Input: part model. Units: mm. Frame: model coordinates. A direction names the side the tool comes from. Round coordinates to 2 decimals unless told otherwise and drop trailing zeros. Order: outer loops, then holes, each group sorted by start corner. A loop starts at its lowest first (then second) coordinate and runs counter-clockwise, first axis right, second up. Notation, with made-up numbers: (-30, 0.25) - (-14, 0.25) arc R18 cw to (-14, 10.25) - close; hole circle Ø10 at (-8, 89.5). An arc over 180 degrees is marked (long way). One line per item, written item: value. Start each with the question number.
from build123d import *

# Parameters (mm, degrees)
SKETCH1_W           = 59
SKETCH1_H           = 68
SKETCH1_R           = 1
SKETCH1_R_2         = 1.5
BOSS_EXTRUDE1_DEPTH = 2
FILLET1_R           = 5
CUT_EXTRUDE1_DEPTH  = 2
SKETCH3_R           = 3
SKETCH3_R_2         = 1
BOSS_EXTRUDE2_DEPTH = 4


with BuildPart() as part:
    # Sketch1 → Boss-Extrude1 (new body)
    with BuildSketch(Plane(origin=(0, 0, 0), x_dir=(1, 0, 0), z_dir=(0, 1, 0))):
        with Locations((29.5, 34)):
            Rectangle(SKETCH1_W, SKETCH1_H)
        with Locations(Location((5, 5, 0), (0, 0, 270))):
            Circle(SKETCH1_R, mode=Mode.SUBTRACT)
        with Locations(Location((54, 5, 0), (0, 0, 270))):
            Circle(SKETCH1_R, mode=Mode.SUBTRACT)
        with Locations(Location((5, 63, 0), (0, 0, 270))):
            Circle(SKETCH1_R, mode=Mode.SUBTRACT)
        with Locations(Location((54, 63, 0), (0, 0, 270))):
            Circle(SKETCH1_R, mode=Mode.SUBTRACT)
        with Locations(Location((9.5, 59, 0), (0, 0, 270))):
            Circle(SKETCH1_R_2, mode=Mode.SUBTRACT)
        with Locations(Location((49.5, 59, 0), (0, 0, 270))):
            Circle(SKETCH1_R_2, mode=Mode.SUBTRACT)
        with Locations(Location((49.5, 9, 0), (0, 0, 270))):
            Circle(SKETCH1_R_2, mode=Mode.SUBTRACT)
        with Locations(Location((9.5, 9, 0), (0, 0, 270))):
            Circle(SKETCH1_R_2, mode=Mode.SUBTRACT)
    extrude(amount=BOSS_EXTRUDE1_DEPTH)

    # Fillet1
    fillet1_edges = [part.edges().sort_by_distance(p)[0] for p in [
        (0, 1, -68),
        (59, 1, -68),
        (59, 1, 0),
        (0, 1, 0),
    ]]
    fillet(fillet1_edges, radius=FILLET1_R)

    # Sketch2 → Cut-Extrude1 (cut)
    with BuildSketch(Plane(origin=(0, 2, 0), x_dir=(1, 0, 0), z_dir=(0, 1, 0))):
        with BuildLine():
            Line((0, 5), (18.940260842, 27.572123903))
            ThreePointArc((18.940260842, 27.572123903), (21.279816411, 34), (18.940260842, 40.427876097))
            Line((18.940260842, 40.427876097), (0, 63))
            Line((0, 63), (0, 5))
        make_face()
        with BuildLine():
            Line((54, 0), (36.255902076, 16.259470082))
            ThreePointArc((36.255902076, 16.259470082), (29.5, 18.886696714), (22.744097924, 16.259470082))
            Line((22.744097924, 16.259470082), (5, 0))
            Line((5, 0), (54, 0))
        make_face()
        with BuildLine():
            Line((54, 68), (5, 68))
            Line((5, 68), (22.744097924, 51.740529918))
            ThreePointArc((22.744097924, 51.740529918), (29.5, 49.113303286), (36.255902076, 51.740529918))
            Line((36.255902076, 51.740529918), (54, 68))
        make_face()
        with BuildLine():
            Line((59, 5), (59, 63))
            Line((59, 63), (40.059739158, 40.427876097))
            ThreePointArc((40.059739158, 40.427876097), (37.720183589, 34), (40.059739158, 27.572123903))
            Line((40.059739158, 27.572123903), (59, 5))
        make_face()
    extrude(amount=-CUT_EXTRUDE1_DEPTH, mode=Mode.SUBTRACT)

    # Sketch3 → Boss-Extrude2 (add)
    # profile 1 of 4: a face of its own
    with BuildSketch(Plane(origin=(0, 2, 0), x_dir=(1, 0, 0), z_dir=(0, 1, 0))):
        with Locations(Location((5, 63, 0), (0, 0, 270))):
            Circle(SKETCH3_R)
        with Locations(Location((5, 63, 0), (0, 0, 270))):
            Circle(SKETCH3_R_2, mode=Mode.SUBTRACT)
    # profile 2 of 4: a face of its own
    with BuildSketch(Plane(origin=(0, 2, 0), x_dir=(1, 0, 0), z_dir=(0, 1, 0))):
        with Locations(Location((54, 63, 0), (0, 0, 90))):
            Circle(SKETCH3_R)
        with Locations(Location((54, 63, 0), (0, 0, 270))):
            Circle(SKETCH3_R_2, mode=Mode.SUBTRACT)
    # profile 3 of 4: a face of its own
    with BuildSketch(Plane(origin=(0, 2, 0), x_dir=(1, 0, 0), z_dir=(0, 1, 0))):
        with Locations(Location((54, 5, 0), (0, 0, 90))):
            Circle(SKETCH3_R)
        with Locations(Location((54, 5, 0), (0, 0, 270))):
            Circle(SKETCH3_R_2, mode=Mode.SUBTRACT)
    # profile 4 of 4: a face of its own
    with BuildSketch(Plane(origin=(0, 2, 0), x_dir=(1, 0, 0), z_dir=(0, 1, 0))):
        with Locations(Location((5, 5, 0), (0, 0, 90))):
            Circle(SKETCH3_R)
        with Locations(Location((5, 5, 0), (0, 0, 270))):
            Circle(SKETCH3_R_2, mode=Mode.SUBTRACT)
    extrude(amount=BOSS_EXTRUDE2_DEPTH)


solid = part.part
1. Line query: line 1 (X direction, y = 4.2, z = -63); line 2 (X direction, y = 0.75, z = -9); line 3 (Y direction, x = 44, z = -50). Output: solid intervals per line, ascending. Write a range as from..to.
2. Section A-A (y = 3.3). Return the cut outline in (x, z).
3. Section C-C (z = -54). Return the cut outline in (x, y), then the cut area to 3 significant figures.
4. Pin query (flat end, axial travel): pin 1 (3.5 mm diameter, centred on x = 9.5, z = -59, fed in from +Y); pin 2 (1.5 mm diameter, centred on x = 43.5, y = 2.5, fed in from -Z). Return the tip coordinate at first contact, or that it passes through.
5. Pull-direction query (X, two-part tool) for faces 1 (the face through (6.8, 4, -2.6)), 2 (the face through (9.34, 1.01, -16.13)), 3 (the face through (53, 6, -4)); classes: released by +X, released by -X, zero draft, split by the parting line, or undercut.
6. Section D-D (x = 43.5). Return the cut outline in (y, z).
7. Set-up query: faces 4 (the face through (9.6, 1.01, -51.56)), 5 (the face through (45.004, 1.014, -59.756)), 6 (the face through (13.996, 1.014, -8.244)), 7 (the face through (51, 4, -5)). Return all of +Z, -Z, +X, -X, +Y, -Y with unobstructed straight access to the full face (end or side cutting, diameter ignored); none if empty.
8. Section B-B (x = 9.5). Return the cut outline in (y, z), then the cut area to 3 significant figures.
Solved:
1. line 1: x = 2..4, 6..8, 51..53, 55..57
1. line 2: x = 3.36..8, 11..14.82, 44.18..48, 51..55.64
1. line 3: y = 0..2
2. outline: circle Ø6 at (5, -63); circle Ø6 at (5, -5); circle Ø6 at (54, -63); circle Ø6 at (54, -5); hole circle Ø2 at (5, -63); hole circle Ø2 at (5, -5); hole circle Ø2 at (54, -63); hole circle Ø2 at (54, -5)
3. outline: (7.55, 0) - (20.28, 0) - (20.28, 2) - (7.55, 2) - close; (38.72, 0) - (51.45, 0) - (51.45, 2) - (38.72, 2) - close
3. area: 50.9 mm²
4. pin 1: stops at y = 2
4. pin 2: stops at z = -58.89
5. face 1: undercut
5. face 2: released by -X
5. face 3: zero draft
6. outline: (0, -58.38) - (2, -58.38) - (2, -44.53) - (0, -44.53) - close; (0, -23.47) - (2, -23.47) - (2, -9.62) - (0, -9.62) - close
7. face 4: -X, +Y, -Y
7. face 5: -Z, +Y, -Y
7. face 6: +Z, +Y, -Y
7. face 7: +Y
8. outline: (0, -63.88) - (2, -63.88) - (2, -60.5) - (0, -60.5) - close; (0, -57.5) - (2, -57.5) - (2, -51.68) - (0, -51.68) - close; (0, -16.32) - (2, -16.32) - (2, -10.5) - (0, -10.5) - close; (0, -7.5) - (2, -7.5) - (2, -4.12) - (0, -4.12) - close
8. area: 36.8 mm²
